```python
from build123d import *

# Parameters (mm, degrees)
SKETCH_1_W          = 65
SKETCH_1_H          = 68
SKETCH_1_R          = 19.1
EXTRUDE_1_DEPTH     = 2
SKETCH_3_W          = 66
SKETCH_3_H          = 2
EXTRUDE_2_DEPTH     = 65
CUT_EXTRUDE_2_DEPTH = 101.056869815
CHAMFER_2_SIZE      = 6
CHAMFER_3_SIZE      = 6
CHAMFER_4_SIZE      = 6
CHAMFER_5_SIZE      = 6
FILLET_1_R          = 2
FILLET_2_R          = 2
SKETCH_5_R          = 2.6
CUT_EXTRUDE_3_DEPTH = 91.629366018


with BuildPart() as part:
    # 草图1 → 凸台-拉伸1 (new body)
    with BuildSketch(Plane.XY):
        with Locations((3.546875, 16.5796875)):
            Rectangle(SKETCH_1_W, SKETCH_1_H)
        with Locations((3.546875, 21.5796875)):
            Circle(SKETCH_1_R, mode=Mode.SUBTRACT)
    extrude(amount=EXTRUDE_1_DEPTH)

    # 草图3 → 凸台-拉伸2 (add)
    with BuildSketch(Plane(origin=(36.046875, 0, 0), x_dir=(0, 0, -1), z_dir=(1, 0, 0))):
        with Locations((33, -16.4203125)):
            Rectangle(SKETCH_3_W, SKETCH_3_H)
    extrude(amount=-EXTRUDE_2_DEPTH)

    # 草图4 → 切除-拉伸2 (cut, through all)
    with BuildSketch(Plane(origin=(0, -15.4203125, 0), x_dir=(1, 0, 0), z_dir=(0, 1, 0))):
        with BuildLine():
            Line((21.446875, 12.59465164), (21.446875, 54.59465164))
            ThreePointArc((21.446875, 54.59465164), (23.546875, 56.69465164), (25.646875, 54.59465164))
            Line((25.646875, 54.59465164), (25.646875, 12.59465164))
            ThreePointArc((25.646875, 12.59465164), (23.546875, 10.49465164), (21.446875, 12.59465164))
        make_face()
        with BuildLine():
            Line((-14.353125, 12.59465164), (-14.353125, 54.59465164))
            ThreePointArc((-14.353125, 54.59465164), (-16.453125, 56.69465164), (-18.553125, 54.59465164))
            Line((-18.553125, 54.59465164), (-18.553125, 12.59465164))
            ThreePointArc((-18.553125, 12.59465164), (-16.453125, 10.49465164), (-14.353125, 12.59465164))
        make_face()
    extrude(amount=-CUT_EXTRUDE_2_DEPTH, mode=Mode.SUBTRACT)

    # 倒角2
    chamfer_2_edges = [part.edges().sort_by_distance(p)[0] for p in [
        (36.046875, -16.4203125, -66),
    ]]
    chamfer(chamfer_2_edges, length=CHAMFER_2_SIZE)

    # 倒角3
    chamfer_3_edges = [part.edges().sort_by_distance(p)[0] for p in [
        (-28.953125, -16.4203125, -66),
    ]]
    chamfer(chamfer_3_edges, length=CHAMFER_3_SIZE)

    # 倒角4
    chamfer_4_edges = [part.edges().sort_by_distance(p)[0] for p in [
        (-28.953125, 50.5796875, 1),
    ]]
    chamfer(chamfer_4_edges, length=CHAMFER_4_SIZE)

    # 倒角5
    chamfer_5_edges = [part.edges().sort_by_distance(p)[0] for p in [
        (36.046875, 50.5796875, 1),
    ]]
    chamfer(chamfer_5_edges, length=CHAMFER_5_SIZE)

    # 圆角1
    fillet_1_edges = [part.edges().sort_by_distance(p)[0] for p in [
        (3.546875, -17.4203125, 2),
    ]]
    fillet(fillet_1_edges, radius=FILLET_1_R)

    # 圆角2
    fillet_2_edges = [part.edges().sort_by_distance(p)[0] for p in [
        (3.546875, -15.4203125, 0),
    ]]
    fillet(fillet_2_edges, radius=FILLET_2_R)

    # 草图5 → 切除-拉伸3 (cut, through all)
    with BuildSketch(Plane(origin=(0, 0, 0), x_dir=(-1, 0, 0), z_dir=(0, 0, -1))):
        with Locations((-27.046875, 45.0796875)):
            Circle(SKETCH_5_R)
        with Locations(Location((19.953125, 45.0796875, 0), (0, 0, 180))):
            Circle(SKETCH_5_R)
        with Locations((19.953125, -1.9203125)):
            Circle(SKETCH_5_R)
        with Locations(Location((-27.046875, -1.9203125, 0), (0, 0, 180))):
            Circle(SKETCH_5_R)
    extrude(amount=-CUT_EXTRUDE_3_DEPTH, mode=Mode.SUBTRACT)


solid = part.part
```
Part model, mm, in its own coordinate system. A direction names the side the tool comes from. Round coordinates to 2 decimals unless told otherwise and drop trailing zeros. Loops run counter-clockwise (first coordinate to the right, second up) from the corner with the lowest first, then second, coordinate; pieces in that order, holes last. Notation, with made-up numbers: (29, 4.5) -> (63, 4.5) arc R20 cw to (63, 18.5) -> close; hole circle Ø5 at (-8.5, 62). An arc over 180 degrees is marked (long way). Use a Markdown table: item, result.
1) Pull direction Z, two halves, no side cores. Call faces 4 (the cylindrical face through (-22.433, -1.139, 0.986)), 5 (the cylindrical face through (23.501, -16.406, -56.694)), 6 (the flat face through (-25.995, -16.434, -62.958)): pulls with the +Z half, pulls with the -Z half, needs draft (parallel to the pull), parting line crosses it, or undercut.
The answers:
| item | result |
|---|---|
| face 4 | needs draft |
| face 5 | undercut |
| face 6 | pulls with the -Z half |
2) Tool access for faces 1 (the cylindrical face through (-0.594, 2.934, 0.986)), 2 (the flat face through (25.647, -16, -34)), 3 (the flat face through (4, -15.42, -34)): list every direction of +Z, -Z, +X, -X, +Y, -Y with a clear straight run to the whole face (end or side of a thin tool).
The answers:
| item | result |
|---|---|
| face 1 | +Z, -Z |
| face 2 | +Y, -Y |
| face 3 | -Z, +X, -X, +Y |
3) Drop flat-ended pins along their axis: pin 1 Ø8 at (x, y) = (14.5, -7.5) entering from -Z; pin 2 Ø19 at (x, z) = (19.5, -49) entering from +Y. Give the stop position or say it passes through.
The answers:
| item | result |
|---|---|
| pin 1 | stops at z = 0 |
| pin 2 | stops at y = -15.42 |
4) Cut at D-D, the plane x = 28.5. List the corners of the cut face in (y, z), and give its area (3 significant figures).
The answers:
| item | result |
|---|---|
| outline | (-17.42, -66) -> (-15.42, -66) -> (-15.42, -2) arc R2 cw to (-13.42, 0) -> (-4.08, 0) -> (-4.08, 2) -> (-15.42, 2) arc R2 ccw to (-17.42, 0) -> close; (0.24, 0) -> (42.92, 0) -> (42.92, 2) -> (0.24, 2) -> close; (47.24, 0) -> (50.58, 0) -> (50.58, 2) -> (47.24, 2) -> close |
| area | 251 mm2 |
5) Cut at A-A, the plane z = -52. List the corners of the cut face in (x, y), and give its area (3 significant figures).
The answers:
| item | result |
|---|---|
| outline | (-28.95, -17.42) -> (-18.55, -17.42) -> (-18.55, -15.42) -> (-28.95, -15.42) -> close; (-14.35, -17.42) -> (21.45, -17.42) -> (21.45, -15.42) -> (-14.35, -15.42) -> close; (25.65, -17.42) -> (36.05, -17.42) -> (36.05, -15.42) -> (25.65, -15.42) -> close |
| area | 113 mm2 |
6) Cut at C-C, the plane y = 37. List the corners of the cut face in (x, z).
The answers:
| item | result |
|---|---|
| outline | (-28.95, 0) -> (-7.72, 0) -> (-7.72, 2) -> (-28.95, 2) -> close; (14.82, 0) -> (36.05, 0) -> (36.05, 2) -> (14.82, 2) -> close |
7) Probe line 1 (Z direction, x = -21, y = 28.5); line 2 (Y direction, x = 13, z = -59). List the from-to ranges inside material, lowest first. Write a range as [from, to].
The answers:
| item | result |
|---|---|
| line 1 | z = [0, 2] |
| line 2 | y = [-17.42, -15.42] |
8) Cut at B-B, the plane x = 17. List the corners of the cut face in (y, z), and give its area (3 significant figures).
The answers:
| item | result |
|---|---|
| outline | (-17.42, -66) -> (-15.42, -66) -> (-15.42, -2) arc R2 cw to (-13.42, 0) -> (8.02, 0) -> (8.02, 2) -> (-15.42, 2) arc R2 ccw to (-17.42, 0) -> close; (35.14, 0) -> (50.58, 0) -> (50.58, 2) -> (35.14, 2) -> close |
| area | 214 mm2 |
